```python
from build123d import *

# Parameters (mm, degrees)
SKETCH1_R           = 30
BOSS_EXTRUDE1_DEPTH = 6.88
SKETCH2_R           = 1.775
CUT_EXTRUDE1_DEPTH  = 7.88
SKETCH3_R           = 5.525
CUT_EXTRUDE2_DEPTH  = 7.88
SKETCH4_R           = 15.5
SKETCH4_R_2         = 5.525
BOSS_EXTRUDE2_DEPTH = 6.88
BOSS_EXTRUDE3_DEPTH = 6.88
FILLET1_R           = 8
BOSS_EXTRUDE4_DEPTH = 6.88
SKETCH8_R           = 3.307099625
CUT_EXTRUDE3_DEPTH  = 7.88
FILLET2_R           = 1
CUT_EXTRUDE4_DEPTH  = 7.8800001
CIRPATTERN7_COUNT   = 5


with BuildPart() as part:
    # Sketch1 → Boss-Extrude1 (new body)
    with BuildSketch(Plane.XY):
        Circle(SKETCH1_R)
    extrude(amount=BOSS_EXTRUDE1_DEPTH)

    # Sketch2 → Cut-Extrude1 (cut, through all)
    with BuildSketch(Plane.XY.offset(6.88)):
        with BuildLine():
            ThreePointArc((-12.74957851, -27.155998376), (-15.133105802, -24.791899388), (-15.484190638, -21.453201167))
            Line((-15.484190638, -21.453201167), (-10.504897898, -0.891395226))
            Line((-10.504897898, -0.891395226), (-18.877603208, 18.537424231))
            ThreePointArc((-18.877603208, 18.537424231), (-19.094099282, 21.887543025), (-17.142995258, 24.619458028))
            ThreePointArc((-17.142995258, 24.619458028), (-29.892573711, -2.536540344), (-12.74957851, -27.155998376))
        make_face()
        with BuildLine():
            ThreePointArc((29.89257372, 2.536540246), (12.74957851, 27.155998377), (-17.142995258, 24.619458028))
            ThreePointArc((-17.142995258, 24.619458028), (-13.90386181, 25.50160376), (-10.836921884, 24.136303033))
            Line((-10.836921884, 24.136303033), (4.480478038, 9.543206057))
            Line((4.480478038, 9.543206057), (25.492681909, 7.079771826))
            ThreePointArc((25.492681909, 7.079771826), (28.502217973, 5.59220348), (29.89257372, 2.536540246))
        make_face()
        with BuildLine():
            ThreePointArc((-6.6150787, -25.617196056), (-9.408118678, -27.479746561), (-12.74957851, -27.155998376))
            ThreePointArc((-12.74957851, -27.155998376), (16.085904462, -25.322789689), (30, 0))
            ThreePointArc((30, 0), (29.973131398, 1.269407029), (29.89257372, 2.536540246))
            ThreePointArc((29.89257372, 2.536540246), (29.905999993, 2.325351424), (29.910478091, 2.113783634))
            ThreePointArc((29.910478091, 2.113783634), (28.913799972, -0.881782076), (26.321112522, -2.683101866))
            Line((26.321112522, -2.683101866), (6.02441986, -8.65181083))
            Line((6.02441986, -8.65181083), (-6.6150787, -25.617196056))
        make_face()
        with Locations((-10.62464872, -22.629998665)):
            Circle(SKETCH2_R)
        with Locations((24.910478091, 2.113783634)):
            Circle(SKETCH2_R)
        with Locations((-14.285829371, 20.51621503)):
            Circle(SKETCH2_R)
    extrude(amount=-CUT_EXTRUDE1_DEPTH, mode=Mode.SUBTRACT)

    # Sketch3 → Cut-Extrude2 (cut, through all)
    with BuildSketch(Plane.XY.offset(6.88)):
        Circle(SKETCH3_R)
    extrude(amount=-CUT_EXTRUDE2_DEPTH, mode=Mode.SUBTRACT)

    # Sketch4 → Boss-Extrude2 (add)
    with BuildSketch(Plane.XY.offset(6.88)):
        Circle(SKETCH4_R)
        Circle(SKETCH4_R_2, mode=Mode.SUBTRACT)
    extrude(amount=-BOSS_EXTRUDE2_DEPTH)

    # Sketch6 → Boss-Extrude3 (add)
    with BuildSketch(Plane.XY.offset(6.88)):
        with BuildLine():
            Line((-5.159411249, 14.616103296), (-29.073470217, 12.586871007))
            Line((-29.073470217, 12.586871007), (-26.536929856, -17.305702703))
            Line((-26.536929856, -17.305702703), (-2.622870888, -15.276470414))
            ThreePointArc((-2.622870888, -15.276470414), (-15.444496417, -1.310545853), (-5.159411249, 14.616103296))
        make_face()
    extrude(amount=-BOSS_EXTRUDE3_DEPTH)

    # Fillet1
    fillet1_edges = [part.edges().sort_by_distance(p)[0] for p in [
        (-26.536929856, -17.305702703, 3.44),
        (-29.073470217, 12.586871007, 3.44),
    ]]
    fillet(fillet1_edges, radius=FILLET1_R)

    # Sketch7 → Boss-Extrude4 (add)
    with BuildSketch(Plane.XY.offset(6.88)):
        with BuildLine():
            Line((13.238211684, 16.431669161), (11.11328194, 11.905669428))
            ThreePointArc((11.11328194, 11.905669428), (4.462352462, 9.504599439), (2.061282474, 16.155528916))
            Line((2.061282474, 16.155528916), (4.186212218, 20.681528649))
            ThreePointArc((4.186212218, 20.681528649), (10.837141695, 23.082598638), (13.238211684, 16.431669161))
        make_face()
        with BuildLine():
            Line((15.817623091, -13.966130451), (12.960457216, -9.862887445))
            ThreePointArc((12.960457216, -9.862887445), (6.000048336, -8.616810313), (4.753971204, -15.577219193))
            Line((4.753971204, -15.577219193), (7.611137078, -19.680462199))
            ThreePointArc((7.611137078, -19.680462199), (14.571545959, -20.926539331), (15.817623091, -13.966130451))
        make_face()
    extrude(amount=-BOSS_EXTRUDE4_DEPTH)

    # Sketch8 → Cut-Extrude3 (cut, through all)
    with BuildSketch(Plane.XY.offset(6.88)):
        with Locations((6.182554141, -17.628840696)):
            Circle(SKETCH8_R)
        with Locations((3.123747346, 18.418528783)):
            Circle(SKETCH8_R)
        with BuildLine():
            Line((11.036190469, -12.786856964), (12.40767393, -14.756476568))
            ThreePointArc((12.40767393, -14.756476568), (12.22076236, -15.8005379), (11.176701028, -15.61362633))
            Line((11.176701028, -15.61362633), (9.805217567, -13.644006726))
            ThreePointArc((9.805217567, -13.644006726), (9.992129137, -12.599945394), (11.036190469, -12.786856964))
        make_face()
        with BuildLine():
            Line((8.723847544, 14.463598968), (9.743846426, 16.636148288))
            ThreePointArc((9.743846426, 16.636148288), (9.383685928, 17.63378771), (8.386046507, 17.273627211))
            Line((8.386046507, 17.273627211), (7.366047624, 15.101077892))
            ThreePointArc((7.366047624, 15.101077892), (7.726208122, 14.10343847), (8.723847544, 14.463598968))
        make_face()
    extrude(amount=-CUT_EXTRUDE3_DEPTH, mode=Mode.SUBTRACT)

    # Fillet2
    fillet2_edges = [part.edges().sort_by_distance(p)[0] for p in [
        (1.777810772, 15.39770726, 3.44),
        (4.346861748, -14.87799694, 3.44),
        (4.588201724, 21.383706907, 3.44),
        (8.125694034, -20.304866722, 3.44),
    ]]
    fillet(fillet2_edges, radius=FILLET2_R)

    # Sketch10 → Cut-Extrude4 (cut, through all)
    with BuildSketch(Plane.XY.offset(6.88)):
        with BuildLine():
            ThreePointArc((-11.874722343, 1.729441895), (-11.957029484, -1.014616145), (-11.413533187, -3.705571507))
            ThreePointArc((-11.413533187, -3.705571507), (-10.153607796, -4.347901647), (-9.511277656, -3.087976256))
            ThreePointArc((-9.511277656, -3.087976256), (-9.964191237, -0.845513454), (-9.895601953, 1.441201579))
            ThreePointArc((-9.895601953, 1.441201579), (-10.74104199, 2.574881932), (-11.874722343, 1.729441895))
        make_face()
    cut_extrude4 = extrude(amount=-CUT_EXTRUDE4_DEPTH, mode=Mode.SUBTRACT)

    # CirPattern7: Cut-Extrude4 ×5 about axis
    cirpattern7_axis = Axis((0, 0, 0), (0, 0, 1))
    for i in range(1, CIRPATTERN7_COUNT):
        add(cut_extrude4.rotate(cirpattern7_axis, i * 360 / CIRPATTERN7_COUNT), mode=Mode.SUBTRACT)


solid = part.part
```
Design review of the part built by this model. Coordinates are the model's own, in mm. A direction names the side the tool comes from. Coordinates: 2 decimals unless noted, no trailing zeros. Order: outer loops, then holes, each group sorted by start corner. A loop starts at its lowest first (then second) coordinate and runs counter-clockwise, first axis right, second up.
1) Take a section at A-A, the plane x = -24. Give the boundary of the cut face in (y, z), and give its area (3 significant figures).
2) Mouldability with a two-part tool opening along X and no side actions: class faces 3 (the cylindrical face through (11.64, 22.61, 3.49)), 4 (the flat face through (14.409, -11.943, 3.488)), 5 (the flat face through (-5, 5, 6.88)) as +X half, -X half, draft (parallel to the pull), parting line (faces both ways), or undercut.
3) Take a section at B-B, the plane z = 4. State how many separate pieces and enclosed holes the cut face has, and give its area (3 significant figures).
4) For faces 1 (the cylindrical face through (10.25, -6.24, 3.49)), 2 (the cylindrical face through (0, 15.5, 3.5)), list the 3-axis set-ups (+Z, -Z, +X, -X, +Y, -Y) from which the entire face can be reached by the end or side of a thin tool; tool diameter is ignored.
5) Clearance check with flat-ended pins moving along their axes: pin 1 (4 mm diameter, centred on x = 24.91, y = 2.11, fed in from +Z); pin 2 (2 mm diameter, centred on x = -1, z = 4, fed in from -Y); pin 3 (1.5 mm diameter, centred on y = -4, z = 4.5, fed in from -X); pin 4 (3 mm diameter, centred on y = -17, z = 5, fed in from +X). State where each tip first meets the part, or that it passes through.
6) Wall thickness on line 1 along Y through (x, z) = (-11, 4.25); line 2 along X through (y, z) = (16.5, 2.25); line 3 along Y through (x, z) = (-1.5, 3.5): over which ranges is each line inside the solid? List them lowest first.
Returned:
1. outline: (-15.09, 0) - (12.45, 0) - (12.45, 6.88) - (-15.09, 6.88) - close
1. area: 189 mm2
2. face 3: undercut
2. face 4: +X half
2. face 5: draft
3. separate pieces: 1
3. enclosed holes: 11
3. area: 1,560 mm2
4. face 1: +Z, -Z
4. face 2: +Z, -Z, +Y
5. pin 1: stops at z = 6.88
5. pin 2: stops at y = -19.42
5. pin 3: stops at x = -27.73
5. pin 4: stops at x = 16.71
6. line 1: y = -27.62 to -24.36, -20.9 to -4.24, 2.58 to 24.28
6. line 2: x = -18 to -2.82, 5.82 to 8.02, 9.68 to 13.27
6. line 3: y = -18.75 to -11.91, -9.89 to -5.32, 5.32 to 9.91, 11.78 to 15.43
